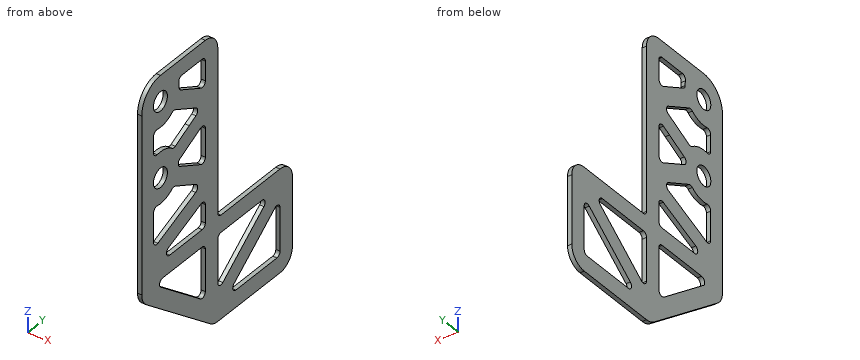
from build123d import *

# Parameters (mm, degrees)
F0_R     = 6.985
F1_DEPTH = 3.175
F3_D     = 14.2748


with BuildPart() as f1:
    # F0 (on Right) → F1 (new body)
    with BuildSketch(Plane.YZ):
        with BuildLine():
            ThreePointArc((38.1, -53.975), (34.3802561211, -44.9947438789), (25.4, -41.275))
            Line((25.4, -41.275), (-34.925, -41.275))
            ThreePointArc((-34.925, -41.275), (-37.1700640303, -40.3450640303), (-38.1, -38.1))
            Line((-38.1, -38.1), (-38.1, 41.275))
            Line((-38.1, 41.275), (-38.1, 47.5751108035))
            Line((-38.1, 47.5751108035), (-38.1, 83.1075017654))
            ThreePointArc((-38.1, 83.1075017654), (-41.8197438789, 92.0877578865), (-50.8, 95.8075017654))
            Line((-50.8, 95.8075017654), (-96.6180321919, 95.8075017654))
            ThreePointArc((-96.6180321919, 95.8075017654), (-110.0884163735, 90.227885947), (-115.6680321919, 76.7575017654))
            Line((-115.6680321919, 76.7575017654), (-115.6680321919, 19.1893243394))
            Line((-115.6680321919, 19.1893243394), (-115.6680321919, -54.4674657519))
            ThreePointArc((-115.6680321919, -54.4674657519), (-114.372733143, -60.0552019855), (-110.7510564099, -64.5031288602))
            Line((-110.7510564099, -64.5031288602), (-45.883024218, -114.8106631083))
            ThreePointArc((-45.883024218, -114.8106631083), (-42.2132151977, -116.7904675622), (-38.1, -117.475))
            Line((-38.1, -117.475), (25.4, -117.475))
            ThreePointArc((25.4, -117.475), (34.3802561211, -113.7552561211), (38.1, -104.775))
            Line((38.1, -104.775), (38.1, -53.975))
        make_face()
        with BuildLine():
            ThreePointArc((-50.8, -88.4454353572), (-52.5780659416, -91.2966105949), (-55.9207560545, -90.9543511342))
            Line((-55.9207560545, -90.9543511342), (-96.2740219927, -59.6589157771))
            ThreePointArc((-96.2740219927, -59.6589157771), (-97.3321328287, -56.1216962006), (-94.3282659382, -53.975))
            Line((-94.3282659382, -53.975), (-53.975, -53.975))
            ThreePointArc((-53.975, -53.975), (-51.7299359697, -54.9049359697), (-50.8, -57.15))
            Line((-50.8, -57.15), (-50.8, -88.4454353572))
        make_face(mode=Mode.SUBTRACT)
        with BuildLine():
            Line((-88.4453191039, -35.1558561059), (-55.1635460576, -21.7200589551))
            ThreePointArc((-55.1635460576, -21.7200589551), (-52.1991915549, -22.0322588212), (-50.8, -24.6642028492))
            Line((-50.8, -24.6642028492), (-50.8, -38.1))
            ThreePointArc((-50.8, -38.1), (-51.7299359697, -40.3450640303), (-53.975, -41.275))
            Line((-53.975, -41.275), (-87.2567730463, -41.275))
            ThreePointArc((-87.2567730463, -41.275), (-90.3735247098, -38.7053792763), (-88.4453191039, -35.1558561059))
        make_face(mode=Mode.SUBTRACT)
        with BuildLine():
            ThreePointArc((-38.1, -57.15), (-37.1700640303, -54.9049359697), (-34.925, -53.975))
            Line((-34.925, -53.975), (6.9827090181, -53.975))
            ThreePointArc((6.9827090181, -53.975), (9.9894060531, -56.1300010097), (8.9145691376, -59.6696312188))
            Line((8.9145691376, -59.6696312188), (-32.9931398805, -91.8012507785))
            ThreePointArc((-32.9931398805, -91.8012507785), (-36.3298076595, -92.1289236249), (-38.1, -89.2816195597))
            Line((-38.1, -89.2816195597), (-38.1, -57.15))
        make_face(mode=Mode.SUBTRACT)
        with BuildLine():
            Line((22.225, -104.775), (-19.6827090181, -104.775))
            ThreePointArc((-19.6827090181, -104.775), (-22.6894060531, -102.6199989903), (-21.6145691376, -99.0803687812))
            Line((-21.6145691376, -99.0803687812), (20.2931398805, -66.9487492215))
            ThreePointArc((20.2931398805, -66.9487492215), (23.6298076595, -66.6210763751), (25.4, -69.4683804403))
            Line((25.4, -69.4683804403), (25.4, -101.6))
            ThreePointArc((25.4, -101.6), (24.4700640303, -103.8450640303), (22.225, -104.775))
        make_face(mode=Mode.SUBTRACT)
        with BuildLine():
            ThreePointArc((-84.8587723654, 5.7476975385), (-83.2201096499, 6.408506351), (-81.481969716, 6.0910896656))
            Line((-81.481969716, 6.0910896656), (-60.3749057725, -4.4348041313))
            ThreePointArc((-60.3749057725, -4.4348041313), (-58.6193026557, -7.4013325865), (-60.6032857265, -10.2202409842))
            Line((-60.6032857265, -10.2202409842), (-99.2394861343, -25.8176116721))
            ThreePointArc((-99.2394861343, -25.8176116721), (-102.203840637, -25.505411806), (-103.6030321919, -22.8734677781))
            Line((-103.6030321919, -22.8734677781), (-103.6030321919, -1.1608908265))
            ThreePointArc((-103.6030321919, -1.1608908265), (-102.4716219082, 1.2689993092), (-99.8837464776, 1.9671082242))
            ThreePointArc((-99.8837464776, 1.9671082242), (-91.969560093, 2.2609528282), (-84.8587723654, 5.7476975385))
        make_face(mode=Mode.SUBTRACT)
        with BuildLine():
            ThreePointArc((-96.8477962041, 27.7163225865), (-91.7608044139, 25.7548199819), (-89.6330321919, 20.7351025284))
            ThreePointArc((-89.6330321919, 20.7351025284), (-91.7608044139, 15.715385075), (-96.8477962041, 13.7538824704))
            ThreePointArc((-96.8477962041, 13.7538824704), (-103.6030321919, 20.7351025284), (-96.8477962041, 27.7163225865))
        make_face(mode=Mode.SUBTRACT)
        with BuildLine():
            Line((-50.8, 31.3570788484), (-50.8, 10.1131262084))
            ThreePointArc((-50.8, 10.1131262084), (-52.304388598, 7.4131849973), (-55.3919260116, 7.2718332496))
            Line((-55.3919260116, 7.2718332496), (-76.6916595751, 17.8938095697))
            ThreePointArc((-76.6916595751, 17.8938095696), (-78.4497335635, 20.7351025284), (-76.6916595751, 23.5763954872))
            Line((-76.6916595751, 23.5763954872), (-61.5697646385, 31.117541927))
            Line((-61.5697646385, 31.117541927), (-55.3919260116, 34.1983718072))
            ThreePointArc((-55.3919260116, 34.1983718072), (-52.304388598, 34.0570200595), (-50.8, 31.3570788484))
        make_face(mode=Mode.SUBTRACT)
        with BuildLine():
            Line((-67.2374686849, 42.4827137621), (-81.481969716, 35.3791153912))
            ThreePointArc((-81.481969716, 35.3791153912), (-83.2201096499, 35.0616987058), (-84.8587723654, 35.7225075184))
            ThreePointArc((-84.8587723654, 35.7225075184), (-91.969560093, 39.2092522286), (-99.8837464776, 39.5030968327))
            ThreePointArc((-99.8837464776, 39.5030968327), (-102.4716219082, 40.2012057477), (-103.6030321919, 42.6310958834))
            Line((-103.6030321919, 42.6310958834), (-103.6030321919, 54.8615084105))
            ThreePointArc((-103.6030321919, 54.8615084105), (-102.4716219082, 57.2913985461), (-99.8837464776, 57.9895074612))
            ThreePointArc((-99.8837464776, 57.9895074612), (-91.969560093, 58.2833520652), (-84.8587723653, 61.7700967755))
            ThreePointArc((-84.8587723654, 61.7700967755), (-83.2201096499, 62.430905588), (-81.481969716, 62.1134889026))
            Line((-81.481969716, 62.1134889026), (-60.3749057725, 51.5875951057))
            ThreePointArc((-60.3749057725, 51.5875951057), (-58.6168317841, 48.7463021469), (-60.3749057725, 45.9050091881))
            Line((-60.3749057725, 45.9050091882), (-67.2374686849, 42.4827137621))
        make_face(mode=Mode.SUBTRACT)
        with Locations((-96.6180321919, 76.7575017654)):
            Circle(F0_R, mode=Mode.SUBTRACT)
        with BuildLine():
            Line((-55.3919260116, 63.2942324866), (-75.8142656696, 73.4786607378))
            ThreePointArc((-75.8142656696, 73.4786607378), (-77.1135956749, 74.6760016746), (-77.5717243057, 76.3824605635))
            ThreePointArc((-77.5717243057, 76.3824605635), (-77.6234503942, 78.209521852), (-77.8500378876, 80.0232160511))
            ThreePointArc((-77.8500378876, 80.0232160511), (-77.1519289726, 82.6110914817), (-74.7220388369, 83.7425017654))
            Line((-74.7220388369, 83.7425017654), (-53.975, 83.7425017654))
            ThreePointArc((-53.975, 83.7425017654), (-51.7299359697, 82.8125657957), (-50.8, 80.5675017654))
            Line((-50.8, 80.5675017654), (-50.8, 66.1355254454))
            ThreePointArc((-50.8, 66.1355254454), (-52.304388598, 63.4355842343), (-55.3919260116, 63.2942324866))
        make_face(mode=Mode.SUBTRACT)
        with Locations((-96.6180321919, 76.7575017654)):
            Circle(F0_R)
    extrude(amount=F1_DEPTH)

    # F3 (through all)
    with Locations(Plane(origin=(0, 0, 0), x_dir=(0, -1, 0), z_dir=(-1, 0, 0))):
        with Locations((96.6180321919, 20.7351025284), (96.6180321919, 76.7575017654)):
            Hole(F3_D / 2)


solid = f1.part
Design review of the part built by this model. Coordinates are the model's own, in mm. Give positions to 0.01 mm unless a question says otherwise; leave off trailing zeros. Order: outer loops, then holes, each group sorted by start corner. A loop starts at its lowest first (then second) coordinate and runs counter-clockwise, first axis right, second up.
1. For pin 1 Ø1 at (x, y) = (1.5, -5.5) entering from +Z (3 decimals); pin 2 Ø1 at (x, z) = (1, -85.5) entering from -Y; pin 3 Ø1.5 at (x, z) = (2, 3) entering from +Y; pin 4 Ø16.5 at (y, z) = (-96.62, 76.76) entering from +X (3 decimals), all flat-tipped, find the tip position at first contact; note any pin that passes through.
Solution:
pin 1: stops at z = -41.275
pin 2: stops at y = -84.32
pin 3: stops at y = -38.1
pin 4: stops at x = 3.175
2. To check wall thickness, follow L1, parallel to Z at x = 2.85, y = -30 (3 decimals); L2, parallel to Z at x = 1.65, y = 2.5 (3 decimals); L3, parallel to Y at x = 2.2, z = -77.5. State the ranges of each line that lie inside material, in increasing order.
Solution:
L1: z = -117.475 to -89.506, -53.975 to -41.275
L2: z = -117.475 to -104.775, -80.591 to -64.588, -53.975 to -41.275
L3: y = -93.99 to -73.27, -50.8 to -38.1, -14.34 to 6.53, 25.4 to 38.1
3. Add section C-C, the plane y = -30. State the section outline as (x, z) points (3 decimals), then the cut area to 3 significant figures.
Solution:
outline: (0, -117.475) - (3.175, -117.475) - (3.175, -89.506) - (0, -89.506) - close; (0, -53.975) - (3.175, -53.975) - (3.175, -41.275) - (0, -41.275) - close
area: 129 mm2
4. Add section D-D, the plane x = 1.25. State how many separate pieces and enclosed holes the cut face has, then the cut area to 3 significant figures.
Solution:
separate pieces: 1
enclosed holes: 10
area: 13,400 mm2
5. Add section A-A, the plane y = 16. State the section outline as (x, z) points (3 decimals), then the cut area to 3 significant figures.
Solution:
outline: (0, -117.475) - (3.175, -117.475) - (3.175, -104.775) - (0, -104.775) - close; (0, -70.24) - (3.175, -70.24) - (3.175, -41.275) - (0, -41.275) - close
area: 132 mm2
6. Add section B-B, the plane y = -3. State the section outline as (x, z) points (3 decimals).
Solution:
outline: (0, -117.475) - (3.175, -117.475) - (3.175, -104.775) - (0, -104.775) - close; (0, -84.808) - (3.175, -84.808) - (3.175, -68.805) - (0, -68.805) - close; (0, -53.975) - (3.175, -53.975) - (3.175, -41.275) - (0, -41.275) - close
